Geometry check sheet. Reference: the model listing, model coordinates, mm. Face numbers are marked on the shaded views. A direction names the side the tool comes from. Round coordinates to 2 decimals unless told otherwise and drop trailing zeros. Loops run counter-clockwise (first coordinate to the right, second up) from the corner with the lowest first, then second, coordinate; pieces in that order, holes last. Notation, with made-up numbers: M 79.25,19.5 L 89.25,19.5 A14 cw 89.25,40.5 Z; hole C -20,17 d5. An arc over 180 degrees is marked long. Use one line per item in the form item = value. Start each with the question number.
1. Material ranges on line 1 (Z direction, x = 489.25, y = 63.5) (1 decimal); line 2 (X direction, y = 56.75, z = -321.31); line 3 (X direction, y = 61.25, z = -321.31), recorded low to high.
2. Set-up check for the marked faces 5 and 6: record each of +Z, -Z, +X, -X, +Y, -Y from which the full face is reachable in a straight line by a thin tool's end or side.
3. Cross-section at C-C (z = -315.5). Record the boundary of the cut face in (x, y) (3 decimals).
4. Cross-section at A-A (z = -321.31). Record the boundary of the cut face in (x, y) (3 decimals), then the cut area to 3 significant figures.
5. Cross-section at D-D (y = 60.5). Record the boundary of the cut face in (x, z) (3 decimals), then the cut area to 3 significant figures.
6. Draft check along X on the marked faces 1, 2, 3 and 4. Enter one of: pulls with the +X half, pulls with the -X half, needs draft (parallel to the pull), parting line crosses it, or undercut.
7. Cross-section at B-B (x = 482.6). Record the boundary of the cut face in (y, z) (3 decimals).
8. Go/stop test with a flat-tipped pin: pin 1 (1.8 mm diameter, centred on x = 489.32, z = -321.31, fed in from -Y). Record where the tip stops, or that it passes through.
```python
from build123d import *

# Parameters (mm, degrees)
BOSS_EXTRUDE1_START             = 47.625
SKETCH5_W                       = 19.785028842
SKETCH5_H                       = 19.785028843
BOSS_EXTRUDE1_DEPTH             = 19.05
F_3_0MM_DOWEL_HOLE1_D           = 3
F_3_0MM_DOWEL_HOLE1_DEPTH       = 25.4
F_3_0MM_DOWEL_HOLE1_CSINK_D     = 3.05
F_3_0MM_DOWEL_HOLE1_CSINK_ANGLE = 90
F_3_0MM_DOWEL_HOLE1_TIP         = 0.901290929
CUT_EXTRUDE1_DEPTH              = 594.535969939


with BuildPart() as part:
    # Sketch5 → Boss-Extrude1 (new body)
    with BuildSketch(Plane(origin=(0, 0, 0), x_dir=(1, 0, 0), z_dir=(0, 1, 0)).offset(BOSS_EXTRUDE1_START)):
        with Locations((482.6, 314.592485579)):
            Rectangle(SKETCH5_W, SKETCH5_H)
    extrude(amount=BOSS_EXTRUDE1_DEPTH)

    # Ø3.0mm Dowel Hole1
    with Locations(Plane(origin=(0, 66.675, 0), x_dir=(1, 0, 0), z_dir=(0, 1, 0))):
        with Locations((475.882485579, 321.31), (489.317514421, 321.31), (489.317514421, 307.874971157), (475.882485579, 307.874971157)):
            CounterSinkHole(F_3_0MM_DOWEL_HOLE1_D / 2, F_3_0MM_DOWEL_HOLE1_CSINK_D / 2, depth=F_3_0MM_DOWEL_HOLE1_DEPTH, counter_sink_angle=F_3_0MM_DOWEL_HOLE1_CSINK_ANGLE)
            with Locations((0, 0, -(F_3_0MM_DOWEL_HOLE1_DEPTH + F_3_0MM_DOWEL_HOLE1_TIP / 2))):  # 118° drill point
                Cone(0, F_3_0MM_DOWEL_HOLE1_D / 2, F_3_0MM_DOWEL_HOLE1_TIP, mode=Mode.SUBTRACT)

    # Sketch8 → Cut-Extrude1 (cut, through all)
    with BuildSketch(Plane.XY):
        with BuildLine():
            ThreePointArc((485.6, 57.15), (481.451949703, 59.921638598), (480.478679656, 55.028679656))
            Line((480.478679656, 55.028679656), (484.721320344, 55.028679656))
            ThreePointArc((484.721320344, 55.028679656), (485.371638598, 56.001949703), (485.6, 57.15))
        make_face()
    extrude(amount=-CUT_EXTRUDE1_DEPTH, mode=Mode.SUBTRACT)


solid = part.part
```
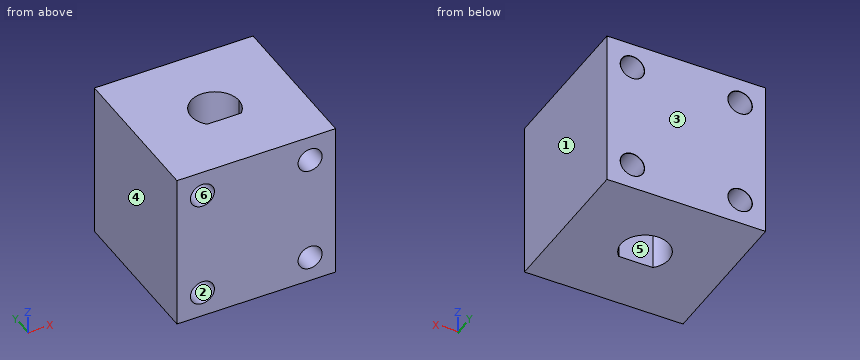
Reported:
q1.line_1 = -324.5 to -322.8, -319.8 to -309.4, -306.4 to -304.7
q1.line_2 = 472.71 to 474.38, 477.38 to 479.63, 485.57 to 487.82, 490.82 to 492.49
q1.line_3 = 472.71 to 474.38, 477.38 to 487.82, 490.82 to 492.49
q2.face_5 = +Z, -Z
q2.face_6 = +Y, -Y
q3.outline = M 472.707,47.625 L 492.493,47.625 L 492.493,66.675 L 472.707,66.675 Z; hole M 480.479,55.029 L 484.721,55.029 A3 ccw long Z
q4.outline = M 472.707,47.625 L 474.382,47.625 L 474.382,66.65 L 474.357,66.675 L 472.707,66.675 Z; M 477.382,47.625 L 487.818,47.625 L 487.818,66.65 L 487.793,66.675 L 477.407,66.675 L 477.382,66.65 Z; M 490.818,47.625 L 492.493,47.625 L 492.493,66.675 L 490.843,66.675 L 490.818,66.65 Z; hole M 480.479,55.029 L 484.721,55.029 A3 ccw long Z
q4.area = 237 mm²
q5.outline = M 472.707,-324.485 L 492.493,-324.485 L 492.493,-304.7 L 472.707,-304.7 Z; hole C 475.882,-321.31 d3; hole C 475.882,-307.875 d3; hole C 489.318,-321.31 d3; hole C 489.318,-307.875 d3
q5.area = 363 mm²
q6.face_1 = pulls with the +X half
q6.face_2 = undercut
q6.face_3 = needs draft
q6.face_4 = pulls with the -X half
q7.outline = M 47.625,-324.485 L 55.029,-324.485 L 55.029,-304.7 L 47.625,-304.7 Z; M 60.15,-324.485 L 66.675,-324.485 L 66.675,-304.7 L 60.15,-304.7 Z
q8.pin_1 = through
